For this review, take the finished solid that the model builds, in its own axes (mm). A direction names the side the tool comes from. Coordinates: 2 decimals unless noted, no trailing zeros. Order: outer loops, then holes, each group sorted by start corner. A loop starts at its lowest first (then second) coordinate and runs counter-clockwise, first axis right, second up. Notation, with made-up numbers: (86.5, -14) -> (130.5, -14) arc R8 ccw to (130.5, -10) -> close; hole circle Ø7 at (-16, 2). An arc over 180 degrees is marked (long way). Return JSON: item names as keys, results as strings. Group by question number.
Item 1: Take a section at A-A (x = 54). Write out the cut boundary in (y, z).
Item 2: Take a section at C-C (z = 3.5). Write out the cut boundary in (x, y), then the cut area to 3 significant figures.
Item 3: Take a section at B-B (y = -43). Write out the cut boundary in (x, z), then the cut area to 3 significant figures.
Item 4: Insertion check: pin 1 (1 mm diameter, centred on x = 23, z = 4.5, fed in from -Y); pin 2 (1.5 mm diameter, centred on x = -43, z = 3, fed in from +Y); pin 3 (4 mm diameter, centred on x = 35.5, y = -55, fed in from +Z). Each pin has a flat end and moves straight along its axis. Give the tip position at first contact, or say it passes through.
Item 5: Draft analysis for pull direction Y (two halves, no side actions). For faces 1 (the flat face through (-42, -62, 3)), 2 (the flat face through (18, -3, 4)), 3 (the flat face through (-46.5, -65, 3)), state which applies: +Y half, -Y half, draft (parallel to the pull), parting line (faces both ways), or undercut.
Item 6: Take a section at D-D (x = 5). Write out the cut boundary in (y, z), then the cut area to 3 significant figures.
Item 7: For line 1 along Y through (x, z) = (8, 12); line 2 along Z through (x, y) = (3, 0); line 3 along Y through (x, z) = (-25.5, 5.25), list the stretches that pass through material, from the lowest coordinate up.
Item 8: Machinability: for faces 4 (the flat face through (59, -48, 3)), 5 (the flat face through (12, -57, 3)), 6 (the flat face through (-44, -41.5, 3)), 7 (the flat face through (-42, -46, 3)), which of the approach directions +Z, -Z, +X, -X, +Y, -Y give a long, thin tool a straight path to every point of the face, cutting with its end or side? Answer none if there is none.
```python
from build123d import *

# Parameters (mm, degrees)
PAD_DEPTH           = 6
CYLINDER001_R       = 5
CYLINDER001_DEPTH   = 6
CYLINDER_R          = 8
CYLINDER_DEPTH      = 6
CUT_PLACEMENT_ANGLE = 90
CHAMFER_SIZE        = 6
CHAMFER001_SIZE     = 6
CHAMFER002_SIZE     = 6
CHAMFER003_SIZE     = 6
CHAMFER004_SIZE     = 3
CHAMFER005_SIZE     = 3
CHAMFER006_SIZE     = 3
CHAMFER007_SIZE     = 3


with BuildPart() as pad:
    # Sketch → Pad (new body)
    with BuildSketch(Plane.XY):
        Polygon((8, 3), (68, 3), (68, -57), (-42, -57), (-42, -66.5), (-48, -66.5), (-48, -41.5), (-42, -41.5), (-42, -51), (62, -51), (62, -3), (8, -3), align=None)
    extrude(amount=PAD_DEPTH)


with BuildPart() as cilindro001:
    # Cylinder001 → Cylinder001 (new body)
    with BuildSketch(Plane(origin=(3, 3, 0), x_dir=(1, 0, 0), z_dir=(0, 0, 1))):
        Circle(CYLINDER001_R)
    extrude(amount=CYLINDER001_DEPTH)


with BuildPart() as chamfer007:
    # Cylinder → Cylinder (new body)
    with BuildSketch(Plane(origin=(3, 3, 0), x_dir=(1, 0, 0), z_dir=(0, 0, 1))):
        Circle(CYLINDER_R)
    extrude(amount=CYLINDER_DEPTH)

    # Cut: cut Cilindro001
    add(cilindro001.part, mode=Mode.SUBTRACT)


with BuildPart() as chamfer007_1:
    # Cut placement: moved
    add(chamfer007.part.moved(Location((0, 3, 3))).rotate(Axis((0, 3, 3), (1, 0, 0)), CUT_PLACEMENT_ANGLE))

    # Fusion: union Pad
    add(pad.part)

    # Chamfer
    chamfer_edges = [chamfer007_1.edges().sort_by_distance(p)[0] for p in [
        (11, 0, 6),
    ]]
    chamfer(chamfer_edges, length=CHAMFER_SIZE)

    # Chamfer001
    chamfer001_edges = [chamfer007_1.edges().sort_by_distance(p)[0] for p in [
        (8.291503, 0, 0),
    ]]
    chamfer(chamfer001_edges, length=CHAMFER001_SIZE)

    # Chamfer002
    chamfer002_edges = [chamfer007_1.edges().sort_by_distance(p)[0] for p in [
        (62, -51, 3),
    ]]
    chamfer(chamfer002_edges, length=CHAMFER002_SIZE)

    # Chamfer003
    chamfer003_edges = [chamfer007_1.edges().sort_by_distance(p)[0] for p in [
        (62, -3, 3),
    ]]
    chamfer(chamfer003_edges, length=CHAMFER003_SIZE)

    # Chamfer004
    chamfer004_edges = [chamfer007_1.edges().sort_by_distance(p)[0] for p in [
        (68, 3, 3),
    ]]
    chamfer(chamfer004_edges, length=CHAMFER004_SIZE)

    # Chamfer005
    chamfer005_edges = [chamfer007_1.edges().sort_by_distance(p)[0] for p in [
        (68, -57, 3),
    ]]
    chamfer(chamfer005_edges, length=CHAMFER005_SIZE)

    # Chamfer006
    chamfer006_edges = [chamfer007_1.edges().sort_by_distance(p)[0] for p in [
        (-48, -66.5, 3),
    ]]
    chamfer(chamfer006_edges, length=CHAMFER006_SIZE)

    # Chamfer007
    chamfer007_edges = [chamfer007_1.edges().sort_by_distance(p)[0] for p in [
        (-48, -41.5, 3),
    ]]
    chamfer(chamfer007_edges, length=CHAMFER007_SIZE)


solid = chamfer007_1.part
```
Findings below:
{
 "1": {"outline": "(-57, 0) -> (-51, 0) -> (-51, 6) -> (-57, 6) -> close; (-3, 0) -> (3, 0) -> (3, 6) -> (-3, 6) -> close"},
 "2": {"outline": "(-48, -63.5) -> (-45, -66.5) -> (-42, -66.5) -> (-42, -57) -> (65, -57) -> (68, -54) -> (68, 0) -> (65, 3) -> (7.33, 3) -> (7.33, -3) -> (56, -3) -> (62, -9) -> (62, -45) -> (56, -51) -> (-42, -51) -> (-42, -41.5) -> (-45, -41.5) -> (-48, -44.5) -> close; (-4.6, -3) -> (-1.33, -3) -> (-1.33, 3) -> (-4.6, 3) -> close", "area": "1,500 mm2"},
 "3": {"outline": "(-46.5, 0) -> (-42, 0) -> (-42, 6) -> (-46.5, 6) -> close; (62, 0) -> (68, 0) -> (68, 6) -> (62, 6) -> close", "area": "63.0 mm2"},
 "4": {"pin 1": "stops at y = -57", "pin 2": "stops at y = -41.5", "pin 3": "stops at z = 6"},
 "5": {"face 1": "draft", "face 2": "undercut", "face 3": "-Y half"},
 "6": {"outline": "(-57, 0) -> (-51, 0) -> (-51, 6) -> (-57, 6) -> close; (-3, -1.59) -> (3, -1.59) -> (3, 1.42) -> (-3, 1.42) -> close; (-3, 10.58) -> (3, 10.58) -> (3, 13.75) -> (-3, 13.75) -> close", "area": "73.0 mm2"},
 "7": {"line 1": "y = -3 to 3", "line 2": "z = -1.93 to 1, 11 to 14", "line 3": "y = -57 to -51"},
 "8": {"face 4": "+Z, -Z", "face 5": "+Z, -Z, +X, -Y", "face 6": "+Z, -Z, -X, +Y", "face 7": "+Z, -Z, +Y"}
}
